```python
from build123d import *

# Parameters (mm, degrees)
CBORE_FOR_M1_6_HEX_HEAD_CAP_SCREW1_D           = 3
CBORE_FOR_M1_6_HEX_HEAD_CAP_SCREW1_CBORE_D     = 5
CBORE_FOR_M1_6_HEX_HEAD_CAP_SCREW1_CBORE_DEPTH = 2
CIRPATTERN1_COUNT                              = 6
F_12_0MM_DOWEL_HOLE1_D                         = 12
F_12_0MM_DOWEL_HOLE1_DEPTH                     = 15
F_12_0MM_DOWEL_HOLE1_TIP                       = 3.605163714
CHAMFER1_SIZE                                  = 2
CIRPATTERN2_COUNT                              = 8


with BuildPart() as part:
    # Sketch1 → Revolve1 (revolve)
    with BuildSketch(Plane(origin=(0, 0, 0), x_dir=(0, 0, -1), z_dir=(1, 0, 0))):
        Polygon((0, 0), (0, 18.5), (52, 18.5), (52, 23.5), (51, 23.5), (51, 25.5), (52, 25.5), (52, 36.5), (49, 36.5), (49, 21.5), (-6, 21.5), (-6, 0), align=None)
    revolve(axis=Axis((0, 0, 6), (0, 0, -1)))

    # CBORE for M1.6 Hex Head Cap Screw1 (through all)
    with Locations(Plane.XY.offset(6)):
        with Locations((15.5, 0)):
            cbore_for_m1_6_hex_head_cap_screw1 = CounterBoreHole(CBORE_FOR_M1_6_HEX_HEAD_CAP_SCREW1_D / 2, CBORE_FOR_M1_6_HEX_HEAD_CAP_SCREW1_CBORE_D / 2, CBORE_FOR_M1_6_HEX_HEAD_CAP_SCREW1_CBORE_DEPTH)

    # CirPattern1: CBORE for M1.6 Hex Head Cap Screw1 ×6 about axis
    cirpattern1_axis = Axis((0, 0, 0), (0, 0, 1))
    for i in range(1, CIRPATTERN1_COUNT):
        add(cbore_for_m1_6_hex_head_cap_screw1.rotate(cirpattern1_axis, i * 360 / CIRPATTERN1_COUNT), mode=Mode.SUBTRACT)

    # Ø12.0mm Dowel Hole1
    with Locations(Plane.XY.offset(6)):
        with Locations((0, -7)):
            Hole(F_12_0MM_DOWEL_HOLE1_D / 2, depth=F_12_0MM_DOWEL_HOLE1_DEPTH)
            with Locations((0, 0, -(F_12_0MM_DOWEL_HOLE1_DEPTH + F_12_0MM_DOWEL_HOLE1_TIP / 2))):  # 118° drill point
                Cone(0, F_12_0MM_DOWEL_HOLE1_D / 2, F_12_0MM_DOWEL_HOLE1_TIP, mode=Mode.SUBTRACT)

    # Chamfer1
    chamfer1_edges = [part.edges().sort_by_distance(p)[0] for p in [
        (0, -21.5, 6),
        (0, -21.5, -49),
        (0, -36.5, -49),
    ]]
    chamfer(chamfer1_edges, length=CHAMFER1_SIZE)

    # Sketch7 → Ø3.0mm Dowel Hole3 (revolve, cut)
    with BuildSketch(Plane(origin=(0, 28, -49), x_dir=(0, -1, 0), z_dir=(1, 0, 0))):
        Polygon((0, 0), (0, 15.901290929), (1.5, 15), (1.5, 0), align=None)
    f_3_0mm_dowel_hole3 = revolve(axis=Axis((0, 28, -42.65), (0, 0, -1)), mode=Mode.SUBTRACT)

    # CirPattern2: Ø3.0mm Dowel Hole3 ×8 about axis
    cirpattern2_axis = Axis((0, 0, 0), (0, 0, 1))
    for i in range(1, CIRPATTERN2_COUNT):
        add(f_3_0mm_dowel_hole3.rotate(cirpattern2_axis, i * 360 / CIRPATTERN2_COUNT), mode=Mode.SUBTRACT)


solid = part.part
```
Model file for the job. Use its own axes, mm. A direction names the side the tool comes from. Give positions to 0.01 mm unless a question says otherwise; leave off trailing zeros. Write each loop counter-clockwise with the first axis right and the second up, starting at its lowest first coordinate (ties: lowest second). Pieces come first, ordered by that corner, then holes. Notation, with made-up numbers: M -5,67.25 L 24,67.25 A8 ccw 24,79.25 Z; hole C -18.75,-22.75 d4. An arc over 180 degrees is marked long. Use a Markdown table: item, result.
1) Pin check, flat tips, straight feed: pin 1 (2.5 mm diameter, centred on x = -15.5, y = 0, fed in from -Z); pin 2 (4.5 mm diameter, centred on x = 15.5, y = 0, fed in from -Z); pin 3 (2 mm diameter, centred on y = 19.5, z = -30.5, fed in from -X); pin 4 (10 mm diameter, centred on x = 21, z = -42, fed in from -Y). Stop position of each tip, or through.
Responses:
| item | result |
|---|---|
| pin 1 | passes through |
| pin 2 | stops at z = 0 |
| pin 3 | stops at x = -10.95 |
| pin 4 | stops at y = -14.36 |
2) Drill centre lines: line 1 (Y direction, x = 7.75, z = 1.2); line 2 (Z direction, x = -13, y = -1); line 3 (Z direction, x = 19, y = -22). Where is each one in solid material? Low to high. Write a range as from..to.
Responses:
| item | result |
|---|---|
| line 1 | y = -20.05..-14.92, -11.92..11.92, 14.92..20.05 |
| line 2 | z = 0..6 |
| line 3 | z = -52..-49 |
3) Cut at A-A (z = -38). List the corners of the cut face in (x, y).
Responses:
| item | result |
|---|---|
| outline | C 0,0 d43; hole C 0,0 d37 |
4) Tool access for faces 4 (the flat face through (-21, -11, -51)), 5 (the cylindrical face through (-0.07, 29.5, -50.48)), 6 (the cylindrical face through (-6.596, 11.205, 5.014)): list every direction of +Z, -Z, +X, -X, +Y, -Y with a clear straight run to the whole face (end or side of a thin tool).
Responses:
| item | result |
|---|---|
| face 4 | -Z |
| face 5 | +Z, -Z |
| face 6 | +Z |
5) Pull direction Y, two halves, no side cores. Call faces 1 (the cylindrical face through (21.286, 19.995, -50.479)), 2 (the conical face through (-33.802, -7.506, -49.125)), 3 (the flat face through (-16, -10, -52)): +Y half, -Y half, draft (parallel to the pull), parting line (faces both ways), or undercut.
Responses:
| item | result |
|---|---|
| face 1 | undercut |
| face 2 | parting line |
| face 3 | draft |
